Part model, mm, in its own coordinate system. Face numbers are marked on the shaded views. A direction names the side the tool comes from. Give positions to 0.01 mm unless a question says otherwise; leave off trailing zeros. Order: outer loops, then holes, each group sorted by start corner. A loop starts at its lowest first (then second) coordinate and runs counter-clockwise, first axis right, second up.
1. Drop flat-ended pins along their axis: pin 1 Ø8 at (y, z) = (61.5, 2.5) entering from +X; pin 2 Ø7 at (x, y) = (147, 49) entering from -Z; pin 3 Ø12 at (x, y) = (24.5, 30) entering from -Z; pin 4 Ø2.5 at (y, z) = (2.5, -14.5) entering from -X. Give the stop position or say it passes through.
2. Mould opens along X. For the marked faces 1, 2 and 3 say: +X half, -X half, draft (parallel to the pull), parting line (faces both ways), or undercut.
3. Slice it at D-D on x = 32.5. List the corners of the cut face in (y, z), and give its area (3 significant figures).
4. Slice it at C-C on z = 2. Give the number of separate pieces and of enclosed holes in the cut face, and give its area (3 significant figures).
5. Which spindle directions (+Z, -Z, +X, -X, +Y, -Y) get a long thin tool onto all of the face, cutting with end or side? Do the marked faces 4 and 5. Say none if no direction does.
6. Slice it at A-A on z = -10. List the corners of the cut face in (x, y) (3 decimals), and give its area (4 significant figures).
7. Probe line 1 (X direction, y = 4, z = -10) (3 decimals); line 2 (Z direction, x = 60, y = 2.7) (3 decimals); line 3 (Y direction, x = 90, z = -8.5). List the from-to ranges inside material, lowest first.
8. Slice it at B-B on x = 139. List the corners of the cut face in (y, z).
from build123d import *

# Parameters (mm, degrees)
SKETCH1_R           = 12.075
BOSS_EXTRUDE1_DEPTH = 10
BOSS_EXTRUDE2_START = -5
SKETCH2_R           = 12.075
SKETCH2_R_2         = 10
BOSS_EXTRUDE2_DEPTH = 5
SKETCH3_W           = 80
SKETCH3_H           = 5
BOSS_EXTRUDE3_DEPTH = 20
SKETCH4_R           = 2.575
CUT_EXTRUDE1_DEPTH  = 174.853386637


with BuildPart() as part:
    # Sketch1 → Boss-Extrude1 (new body)
    with BuildSketch(Plane.XY):
        with BuildLine():
            Line((134.231894093, 70), (145, 70))
            ThreePointArc((145, 70), (155.606601718, 65.606601718), (160, 55))
            Line((160, 55), (160, 42))
            ThreePointArc((160, 42), (147.69848481, 12.30151519), (118, 0))
            Line((118, 0), (42, 0))
            ThreePointArc((42, 0), (12.30151519, 12.30151519), (0, 42))
            Line((0, 42), (0, 55))
            ThreePointArc((0, 55), (4.393398282, 65.606601718), (15, 70))
            Line((15, 70), (25.768105907, 70))
            ThreePointArc((25.768105907, 70), (32.276192497, 67.592417858), (35.650528477, 61.528961786))
            add(Edge.make_bspline(
                [(35.650528477, 61.528961786), (42.075693473, 20), (80, 20), (117.924306527, 20), (124.349471523, 61.528961786)],
                knots=[4.882630888, 4.882630888, 4.882630888, 6.283185307, 6.283185307, 7.683739727, 7.683739727, 7.683739727], degree=2, weights=[1, 0.764663574, 1, 0.764663574, 1]))
            ThreePointArc((124.349471523, 61.528961786), (127.723807503, 67.592417858), (134.231894093, 70))
        make_face()
        with Locations((19, 50)):
            Circle(SKETCH1_R, mode=Mode.SUBTRACT)
        with Locations(Location((141, 50, 0), (0, 0, 180))):
            Circle(SKETCH1_R, mode=Mode.SUBTRACT)
    extrude(amount=BOSS_EXTRUDE1_DEPTH)

    # Sketch2 → Boss-Extrude2 (add)
    # profile 1 of 2: a face of its own
    with BuildSketch(Plane.XY.offset(10).offset(BOSS_EXTRUDE2_START)):
        with Locations(Location((141, 50, 0), (0, 0, 180))):
            Circle(SKETCH2_R)
        with Locations((141, 50)):
            Circle(SKETCH2_R_2, mode=Mode.SUBTRACT)
    # profile 2 of 2: a face of its own
    with BuildSketch(Plane.XY.offset(10).offset(BOSS_EXTRUDE2_START)):
        with Locations((19, 50)):
            Circle(SKETCH2_R)
        with Locations((19, 50)):
            Circle(SKETCH2_R_2, mode=Mode.SUBTRACT)
    extrude(amount=BOSS_EXTRUDE2_DEPTH)

    # Sketch3 → Boss-Extrude3 (add)
    with BuildSketch(Plane(origin=(0, 0, 0), x_dir=(-1, 0, 0), z_dir=(0, 0, -1))):
        with Locations((-80, 2.5)):
            Rectangle(SKETCH3_W, SKETCH3_H)
    extrude(amount=BOSS_EXTRUDE3_DEPTH)

    # Sketch4 → Cut-Extrude1 (cut, through all)
    with BuildSketch(Plane(origin=(0, 5, 0), x_dir=(1, 0, 0), z_dir=(0, 1, 0))):
        with Locations(Location((100, 10, 0), (0, 0, 270))):
            Circle(SKETCH4_R)
        with Locations(Location((60, 10, 0), (0, 0, 90))):
            Circle(SKETCH4_R)
    extrude(amount=-CUT_EXTRUDE1_DEPTH, mode=Mode.SUBTRACT)


solid = part.part
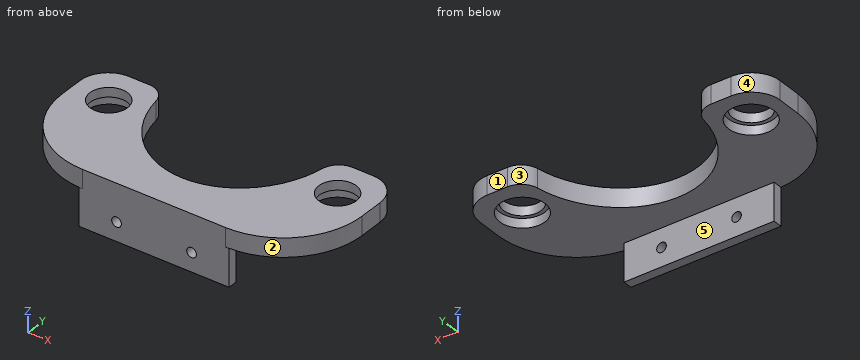
Data:
1. pin 1: stops at x = 159.79
1. pin 2: passes through
1. pin 3: stops at z = 0
1. pin 4: stops at x = 40
2. face 1: draft
2. face 2: +X half
2. face 3: undercut
3. outline: (1.09, 0) - (67.39, 0) - (67.39, 10) - (1.09, 10) - close
3. area: 663 mm2
4. separate pieces: 1
4. enclosed holes: 2
4. area: 5,860 mm2
5. face 4: +Z, -Z, -X, +Y
5. face 5: -Z, +X, -X, +Y
6. outline: (40, 0) - (57.425, 0) - (57.425, 5) - (40, 5) - close; (62.575, 0) - (97.425, 0) - (97.425, 5) - (62.575, 5) - close; (102.575, 0) - (120, 0) - (120, 5) - (102.575, 5) - close
6. area: 348.5 mm2
7. line 1: x = 40 to 57.425, 62.575 to 97.425, 102.575 to 120
7. line 2: z = -20 to -12.575, -7.425 to 10
7. line 3: y = 0 to 5
8. outline: (5.63, 0) - (38.09, 0) - (38.09, 5) - (40.2, 5) - (40.2, 10) - (5.63, 10) - close; (59.8, 5) - (61.91, 5) - (61.91, 0) - (70, 0) - (70, 10) - (59.8, 10) - close
